from build123d import *

# Parameters (mm, degrees)
F0_W      = 705
F0_H      = 480
F1_DEPTH  = 690
F4_T      = -2.54
F5_DEPTH  = 705
F2_W      = 705
F2_H      = 250
F6_DEPTH  = 2.54
F7_W      = 699.92
F7_H      = 2.54
F8_DEPTH  = 265
F9_W      = 40
F9_H      = 40
F9_W_2    = 30
F9_H_2    = 30
F10_DEPTH = 865
F11_W     = 699.92
F11_H     = 225
F12_DEPTH = 2.54


with BuildPart() as f1:
    # F0 (on Front) → F1 (new body)
    with BuildSketch(Plane.XZ):
        Rectangle(F0_W, F0_H)
    extrude(amount=F1_DEPTH)

    # F4
    f4_openings = [f1.faces().sort_by_distance(p)[0] for p in [
        (0, -345, 240),
    ]]
    offset(amount=F4_T, openings=f4_openings)

    # F3 (on face) → F5 (cut, through all)
    with BuildSketch(Plane.YZ.offset(352.5)):
        Polygon((-690, -240), (-250, 240), (-690, 240), align=None)
    extrude(amount=-F5_DEPTH, mode=Mode.SUBTRACT)

    # F2 (on face) → F6 (join)
    with BuildSketch(Plane.XY.offset(240)):
        with Locations((0, -125)):
            Rectangle(F2_W, F2_H)
    extrude(amount=F6_DEPTH)

    # F7 (on face) → F8 (join)
    with BuildSketch(Plane(origin=(0, 0, 240), x_dir=(1, 0, 0), z_dir=(0, 0, -1))):
        with Locations((0, 248.73)):
            Rectangle(F7_W, F7_H)
    extrude(amount=F8_DEPTH)

    # F9 (on face) → F10 (join)
    with BuildSketch(Plane(origin=(0, 0, -240), x_dir=(1, 0, 0), z_dir=(0, 0, -1))):
        with Locations((-332.5, 670)):
            Rectangle(F9_W, F9_H)
        with Locations((-332.5, 670)):
            Rectangle(F9_W_2, F9_H_2, mode=Mode.SUBTRACT)
        with Locations((-332.5, 20)):
            Rectangle(F9_W, F9_H)
        with Locations((-332.5, 20)):
            Rectangle(F9_W_2, F9_H_2, mode=Mode.SUBTRACT)
        with Locations((332.5, 20)):
            Rectangle(F9_W, F9_H)
        with Locations((332.5, 20)):
            Rectangle(F9_W_2, F9_H_2, mode=Mode.SUBTRACT)
        with Locations((332.5, 670)):
            Rectangle(F9_W, F9_H)
        with Locations((332.5, 670)):
            Rectangle(F9_W_2, F9_H_2, mode=Mode.SUBTRACT)
    extrude(amount=F10_DEPTH)

    # F11 (on face) → F12 (join)
    with BuildSketch(Plane.XY.offset(-237.46)):
        with Locations((0, -799.96)):
            Rectangle(F11_W, F11_H)
    extrude(amount=-F12_DEPTH)


solid = f1.part
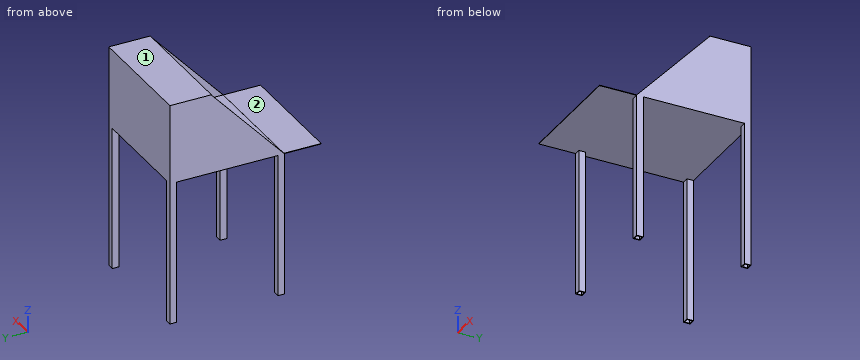
Source: CAD feature listing. Evaluate the final solid. Frame: model axes, mm. Face numbers are marked on the shaded views. A direction names the side the tool comes from. Round coordinates to 2 decimals unless told otherwise and drop trailing zeros. Write each loop counter-clockwise with the first axis right and the second up, starting at its lowest first coordinate (ties: lowest second). Pieces come first, ordered by that corner, then holes. Notation, with made-up numbers: (-21, 60.25) - (14, 60.25) arc R15 ccw to (14, 75.25) - close; hole circle Ø2 at (69, -26). An arc over 180 degrees is marked (long way). Use CSV: the item, a comma, the result in double quotes. Start each with the question number.
(1) First-contact query: pin 1 Ø3 at (y, z) = (-772, -238.5) entering from -X; pin 2 Ø2 at (x, y) = (-163.5, -805.5) entering from +Z; pin 3 Ø1.3 at (y, z) = (-797.5, -239) entering from +X. Flat tips, straight axial feed; report the tip coordinate or a pass-through.
(2) Set-up query: the marked faces 1 and 2. Return all of +Z, -Z, +X, -X, +Y, -Y with unobstructed straight access to the full face (end or side cutting, diameter ignored); none if empty.
(3) Cut plane B-B, the plane y = -111. Return loops of the section in (x, z).
(4) Cut plane D-D, the plane x = -139. Return loops of the section in (y, z), and give its area (3 significant figures).
(5) Cut plane C-C, the plane z = 51. Return loops of the section in (x, y).
(6) Material intervals for probe 1 along X at (y, z) = (-669, -705); probe 2 along X at (y, z) = (-63.5, -139); probe 3 along Y at (x, z) = (288.5, 131), sorted ascending. Write a range as [from, to].
(7) Cut plane A-A, the plane z = -686. Give the number of separate pieces and of enclosed holes in the cut face, and give its area (3 significant figures).
Geometry says:
1,pin 1,"x = -349.96"
1,pin 2,"z = -237.46"
1,pin 3,"x = 349.96"
2,face 1,"+Z, +X, -X, +Y, -Y"
2,face 2,"+Z, +X, -X, -Y"
3,outline,"(-352.5, -240) - (352.5, -240) - (352.5, 242.54) - (-352.5, 242.54) - close; hole (-349.96, -237.46) - (349.96, -237.46) - (349.96, 240) - (-349.96, 240) - close"
4,outline,"(-912.46, -240) - (0, -240) - (0, 242.54) - (-250, 242.54) - (-250, -25) - (-247.46, -25) - (-247.46, 240) - (-2.54, 240) - (-2.54, -237.46) - (-687.46, -237.46) - (-687.46, -237.23) - (-687.67, -237.46) - (-912.46, -237.46) - close"
4,area,"4,840 mm²"
5,outline,"(-352.5, -423.25) - (-349.96, -423.25) - (-349.96, -250) - (349.96, -250) - (349.96, -423.25) - (352.5, -423.25) - (352.5, 0) - (-352.5, 0) - close; hole (-349.96, -247.46) - (349.96, -247.46) - (349.96, -2.54) - (-349.96, -2.54) - close"
6,probe 1,"[-352.5, -347.5], [-317.5, -312.5], [312.5, 317.5], [347.5, 352.5]"
6,probe 2,"[-352.5, -349.96], [349.96, 352.5]"
6,probe 3,"[-250, -247.46], [-2.54, 0]"
7,separate pieces,"4"
7,enclosed holes,"4"
7,area,"2,800 mm²"
